```python
from build123d import *

# Parameters (mm, degrees)
SKETCH1_W           = 50
SKETCH1_H           = 60
BOSS_EXTRUDE1_DEPTH = 25
CUT_EXTRUDE1_START  = -10
SKETCH2_R           = 22.5
CUT_EXTRUDE1_DEPTH  = 30
SKETCH3_R           = 7.5
CUT_EXTRUDE2_DEPTH  = 64.442887702
SKETCH4_R           = 10
CUT_EXTRUDE3_DEPTH  = 10
SKETCH10_W          = 11
SKETCH10_H          = 10
CUT_EXTRUDE9_DEPTH  = 11
SKETCH11_R          = 2.25
CUT_EXTRUDE10_DEPTH = 50.398886748
SKETCH12_R          = 2
CUT_EXTRUDE11_DEPTH = 50.371044201
SKETCH13_R          = 3.5
CUT_EXTRUDE12_DEPTH = 50.371044201
CHAMFER1_SIZE       = 3
FILLET1_R           = 4
SKETCH14_R          = 2
CUT_EXTRUDE13_DEPTH = 10
CUT_EXTRUDE14_DEPTH = 3
BOSS_EXTRUDE2_DEPTH = 5
CHAMFER2_SIZE       = 3
FILLET2_R           = 1


with BuildPart() as part:
    # Sketch1 → Boss-Extrude1 (new body)
    with BuildSketch(Plane(origin=(0, 0, 0), x_dir=(1, 0, 0), z_dir=(0, 1, 0))):
        Rectangle(SKETCH1_W, SKETCH1_H)
    extrude(amount=BOSS_EXTRUDE1_DEPTH)

    # Sketch2 → Cut-Extrude1 (cut)
    with BuildSketch(Plane.ZY.offset(25).offset(CUT_EXTRUDE1_START)):
        with Locations((0, 25)):
            Circle(SKETCH2_R)
    extrude(amount=-CUT_EXTRUDE1_DEPTH, mode=Mode.SUBTRACT)

    # Sketch3 → Cut-Extrude2 (cut, through all)
    with BuildSketch(Plane.ZY.offset(25)):
        with Locations((0, 25)):
            Circle(SKETCH3_R)
    extrude(amount=-CUT_EXTRUDE2_DEPTH, mode=Mode.SUBTRACT)

    # Sketch4 → Cut-Extrude3 (cut)
    with BuildSketch(Plane.XY.offset(30)):
        with Locations((0, 25)):
            Circle(SKETCH4_R)
    extrude(amount=-CUT_EXTRUDE3_DEPTH, mode=Mode.SUBTRACT)

    # Sketch10 → Cut-Extrude9 (cut)
    with BuildSketch(Plane(origin=(25, 0, 0), x_dir=(0, 0, -1), z_dir=(1, 0, 0))):
        with Locations((-10, 5)):
            Rectangle(SKETCH10_W, SKETCH10_H)
        with Locations((10, 5)):
            Rectangle(SKETCH10_W, SKETCH10_H)
    cut_extrude9 = extrude(amount=-CUT_EXTRUDE9_DEPTH, mode=Mode.SUBTRACT)

    # Sketch11 → Cut-Extrude10 (cut, symmetric)
    with BuildSketch(Plane(origin=(0, 0, -4.5), x_dir=(-1, 0, 0), z_dir=(0, 0, -1))):
        with Locations(Location((-21, 5, 0), (0, 0, 90))):
            Circle(SKETCH11_R)
    cut_extrude10 = extrude(amount=CUT_EXTRUDE10_DEPTH, both=True, mode=Mode.SUBTRACT)

    # Mirror1: Cut-Extrude9, Cut-Extrude10 across plane
    add(cut_extrude9.mirror(Plane(origin=(0, 0, 0), x_dir=(0, 0, 1), z_dir=(1, 0, 0))), mode=Mode.SUBTRACT)
    add(cut_extrude10.mirror(Plane(origin=(0, 0, 0), x_dir=(0, 0, 1), z_dir=(1, 0, 0))), mode=Mode.SUBTRACT)

    # Sketch12 → Cut-Extrude11 (cut, symmetric)
    with BuildSketch(Plane(origin=(0, -2.5, 2.5), x_dir=(1, 0, 0), z_dir=(0, -0.7071067811865475, 0.7071067811865477))):
        with Locations(Location((20, 33.890872965, 0), (0, 0, 270))):
            Circle(SKETCH12_R)
        with Locations(Location((-20, 33.890872965, 0), (0, 0, 270))):
            Circle(SKETCH12_R)
    cut_extrude11 = extrude(amount=CUT_EXTRUDE11_DEPTH, both=True, mode=Mode.SUBTRACT)

    # Sketch13 → Cut-Extrude12 (cut, through all)
    with BuildSketch(Plane(origin=(0, -2.5, 2.5), x_dir=(1, 0, 0), z_dir=(0, -0.7071067811865475, 0.7071067811865477))):
        with Locations(Location((-20, 33.890872965, 0), (0, 0, 90))):
            Circle(SKETCH13_R)
        with Locations(Location((20, 33.890872965, 0), (0, 0, 90))):
            Circle(SKETCH13_R)
    cut_extrude12 = extrude(amount=CUT_EXTRUDE12_DEPTH, mode=Mode.SUBTRACT)

    # Mirror3: Cut-Extrude11, Cut-Extrude12 across plane
    add(cut_extrude11.mirror(Plane.XY), mode=Mode.SUBTRACT)
    add(cut_extrude12.mirror(Plane.XY), mode=Mode.SUBTRACT)

    # Chamfer1
    # the kernel refuses this chamfer: 3 mm, written as the material it takes off along each edge
    with BuildSketch(Plane(origin=(25, -7.715048964, -30), x_dir=(-0.9996219169112965, 0, -0.02749587661058676), z_dir=(0, 1, 0))) as chamfer1_piece_1:
        Polygon((CHAMFER1_SIZE * 0.999621916911, CHAMFER1_SIZE * 0.0274958766106), (-CHAMFER1_SIZE * 0.0274958766106, CHAMFER1_SIZE * 0.999621916911), (0, 0), align=None)
    extrude(amount=40.430097928, mode=Mode.SUBTRACT)
    with BuildSketch(Plane(origin=(-25, -7.715048964, -30), x_dir=(0.9996219169112965, 0, -0.02749587661058676), z_dir=(0, 1, 0))) as chamfer1_piece_2:
        Polygon((CHAMFER1_SIZE * 0.999621916911, -CHAMFER1_SIZE * 0.0274958766106), (-CHAMFER1_SIZE * 0.0274958766106, -CHAMFER1_SIZE * 0.999621916911), (0, 0), align=None)
    extrude(amount=40.430097928, mode=Mode.SUBTRACT)

    # Fillet1
    fillet1_edges = [part.edges().sort_by_distance(p)[0] for p in [
        (-25, 10, 10),
        (-25, 10, -10),
        (25, 10, 10),
        (25, 10, -10),
    ]]
    fillet(fillet1_edges, radius=FILLET1_R)

    # Sketch14 → Cut-Extrude13 (cut)
    with BuildSketch(Plane.XZ):
        with Locations(Location((-15, -20.205680561, 0), (0, 0, 270))):
            Circle(SKETCH14_R)
        with Locations(Location((15, -20.205680561, 0), (0, 0, 270))):
            Circle(SKETCH14_R)
    extrude(amount=-CUT_EXTRUDE13_DEPTH, mode=Mode.SUBTRACT)

    # Sketch15 → Cut-Extrude14 (cut)
    with BuildSketch(Plane.XY.offset(30)):
        Polygon((-21, 0.958548116), (-17.5, 2.979274058), (-17.5, 7.020725942), (-21, 9.041451884), (-24.5, 7.020725942), (-24.5, 2.979274058), align=None)
        Polygon((21, 0.958548116), (24.5, 2.979274058), (24.5, 7.020725942), (21, 9.041451884), (17.5, 7.020725942), (17.5, 2.979274058), align=None)
    extrude(amount=-CUT_EXTRUDE14_DEPTH, mode=Mode.SUBTRACT)

    # Sketch16 → Boss-Extrude2 (add)
    with BuildSketch(Plane.XY.offset(30)):
        with BuildLine():
            Line((-25, 9.464101615), (-27, 6))
            Line((-27, 6), (-27, 0))
            ThreePointArc((-27, 0), (-26.414213562, -1.414213562), (-25, -2))
            Line((-25, -2), (-19, -2))
            Line((-19, -2), (-15.535898385, 0))
            Line((-15.535898385, 0), (-25, 0))
            Line((-25, 0), (-25, 9.464101615))
        make_face()
    boss_extrude2 = extrude(amount=-BOSS_EXTRUDE2_DEPTH)

    # Mirror4: Boss-Extrude2 across plane
    add(boss_extrude2.mirror(Plane(origin=(0, 0, 0), x_dir=(0, 0, 1), z_dir=(1, 0, 0))))

    # Chamfer2
    # the kernel refuses this chamfer: 3 mm, written as the material it takes off along each edge
    with BuildSketch(Plane(origin=(-25, 0, 25), x_dir=(0.9996219169112968, -0.02749587661058636, 0), z_dir=(0, 0, -1))) as chamfer2_piece_1:
        Polygon((CHAMFER2_SIZE * 0.999621916911, -CHAMFER2_SIZE * 0.0274958766106), (-CHAMFER2_SIZE * 0.0274958766106, -CHAMFER2_SIZE * 0.999621916911), (0, 0), align=None)
    extrude(amount=17.215048964, mode=Mode.SUBTRACT)
    with BuildSketch(Plane(origin=(-25, 0, 12.215048964), x_dir=(0.9996219169112968, -0.02749587661058636, 0), z_dir=(0, 0, -1))) as chamfer2_piece_2:
        Polygon((CHAMFER2_SIZE * 0.999621916911, -CHAMFER2_SIZE * 0.0274958766106), (-CHAMFER2_SIZE * 0.0274958766106, -CHAMFER2_SIZE * 0.999621916911), (0, 0), align=None)
    extrude(amount=24.430097928, mode=Mode.SUBTRACT)
    with BuildSketch(Plane(origin=(-25, 0, -7.784951036), x_dir=(0.9996219169112968, -0.02749587661058636, 0), z_dir=(0, 0, -1))) as chamfer2_piece_3:
        Polygon((CHAMFER2_SIZE * 0.999621916911, -CHAMFER2_SIZE * 0.0274958766106), (-CHAMFER2_SIZE * 0.0274958766106, -CHAMFER2_SIZE * 0.999621916911), (0, 0), align=None)
    extrude(amount=26.930097928, mode=Mode.SUBTRACT)
    with BuildSketch(Plane(origin=(-16.54463656, 0, -35.45536344), x_dir=(0.7068394360709561, -0.027495876610586396, 0.7068394360703909), z_dir=(-0.7071067811862648, 0, 0.7071067811868302))) as chamfer2_piece_4:
        Polygon((CHAMFER2_SIZE * 0.999621916911, CHAMFER2_SIZE * 0.0274958766106), (-CHAMFER2_SIZE * 0.0274958766106, CHAMFER2_SIZE * 0.999621916911), (0, 0), align=None)
    extrude(amount=19.672738615, mode=Mode.SUBTRACT)
    with BuildSketch(Plane(origin=(-29.715048964, 0, -30), x_dir=(0, -0.02749587661058636, 0.9996219169112968), z_dir=(1, 0, 0))) as chamfer2_piece_5:
        Polygon((CHAMFER2_SIZE * 0.999621916911, -CHAMFER2_SIZE * 0.0274958766106), (-CHAMFER2_SIZE * 0.0274958766106, -CHAMFER2_SIZE * 0.999621916911), (0, 0), align=None)
    extrude(amount=59.430097928, mode=Mode.SUBTRACT)
    with BuildSketch(Plane(origin=(16.54463656, 0, -35.45536344), x_dir=(-0.7068394360709561, -0.027495876610586396, 0.7068394360703909), z_dir=(0.7071067811862648, 0, 0.7071067811868302))) as chamfer2_piece_6:
        Polygon((CHAMFER2_SIZE * 0.999621916911, -CHAMFER2_SIZE * 0.0274958766106), (-CHAMFER2_SIZE * 0.0274958766106, -CHAMFER2_SIZE * 0.999621916911), (0, 0), align=None)
    extrude(amount=19.672738615, mode=Mode.SUBTRACT)
    with BuildSketch(Plane(origin=(25, 0, -34.715048964), x_dir=(0.027495876610586778, 0.9996219169112968, 0), z_dir=(0, 0, 1))) as chamfer2_piece_7:
        Polygon((CHAMFER2_SIZE * 0.999621916911, CHAMFER2_SIZE * 0.0274958766106), (-CHAMFER2_SIZE * 0.0274958766106, CHAMFER2_SIZE * 0.999621916911), (0, 0), align=None)
    extrude(amount=26.930097928, mode=Mode.SUBTRACT)
    with BuildSketch(Plane(origin=(25, 0, 7.784951036), x_dir=(0.027495876610586778, 0.9996219169112968, 0), z_dir=(0, 0, 1))) as chamfer2_piece_8:
        Polygon((CHAMFER2_SIZE * 0.999621916911, CHAMFER2_SIZE * 0.0274958766106), (-CHAMFER2_SIZE * 0.0274958766106, CHAMFER2_SIZE * 0.999621916911), (0, 0), align=None)
    extrude(amount=17.215048964, mode=Mode.SUBTRACT)
    with BuildSketch(Plane(origin=(25, 0, -12.215048964), x_dir=(0.027495876610586778, 0.9996219169112968, 0), z_dir=(0, 0, 1))) as chamfer2_piece_9:
        Polygon((CHAMFER2_SIZE * 0.999621916911, CHAMFER2_SIZE * 0.0274958766106), (-CHAMFER2_SIZE * 0.0274958766106, CHAMFER2_SIZE * 0.999621916911), (0, 0), align=None)
    extrude(amount=24.430097928, mode=Mode.SUBTRACT)

    # Fillet2
    fillet2_edges = [part.edges().sort_by_distance(p)[0] for p in [
        (-18.767949192, 0, 25),
        (18.767949192, 0, 25),
        (-25, 6.232050808, 25),
        (25, 6.232050808, 25),
        (-23.5, 1.5, 25),
        (23.5, 1.5, 25),
    ]]
    fillet(fillet2_edges, radius=FILLET2_R)


solid = part.part
```
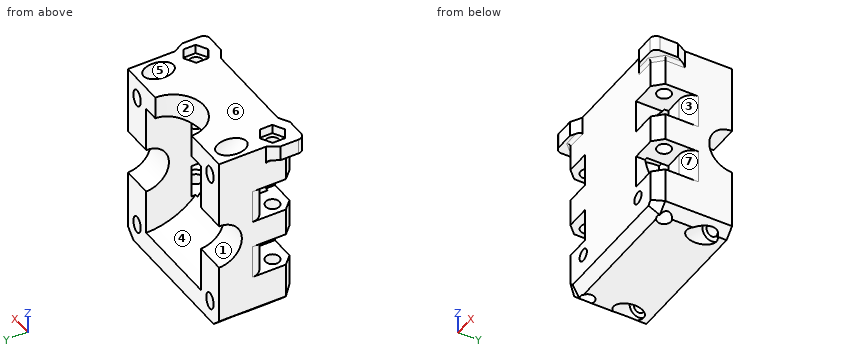
Check sheet for the modelled part. Datum: model origin and axes. Units: mm. Face numbers are marked on the shaded views. A direction names the side the tool comes from. Give positions to 0.01 mm unless a question says otherwise; leave off trailing zeros. Order: outer loops, then holes, each group sorted by start corner. A loop starts at its lowest first (then second) coordinate and runs counter-clockwise, first axis right, second up. Notation, with made-up numbers: M 20,79.5 L 76,79.5 A18 cw 76,94.5 Z; hole C 50,-33.75 d10. An arc over 180 degrees is marked long. Answer in a Markdown table with one row per item.
1) Cross-section at D-D, the plane y = 5. Count the separate pieces of the cut face and the enclosed holes in it, plus the area to 3 significant figures.
Filled sheet:
| item | result |
|---|---|
| separate pieces | 10 |
| enclosed holes | 2 |
| area | 1,550 mm2 |
2) Gauge pin test, flat ends, axial feed: P1, Ø4, axis at x = 21, y = 5, coming from the +Z side; P2, Ø8, axis at y = 9.5, z = -22, coming from the +X side; P3, Ø5, axis at x = -17, z = -8, coming from the -Y side; P4, Ø5.5, axis at x = -20.5, y = 4.5, coming from the +Z side. Record the tip position at first contact, or that the pin passes through.
Filled sheet:
| item | result |
|---|---|
| P1 | passes through |
| P2 | stops at x = 25 |
| P3 | stops at y = 10 |
| P4 | stops at z = 27 |
3) Cross-section at B-B, the plane z = -14.5. Enter the section's corners in (x, y), plus the area to 3 significant figures.
Filled sheet:
| item | result |
|---|---|
| outline | M -25,14 A4 ccw -21,10 L -15,10 L -15,25 L -25,25 Z; M -14,0 L 14,0 L 14,7.8 L -14,7.8 Z; M 15,10 L 21,10 A4 ccw 25,14 L 25,25 L 15,25 Z |
| area | 511 mm2 |
4) Cross-section at A-A, the plane x = 0. Enter the section's corners in (y, z), plus the area to 3 significant figures.
Filled sheet:
| item | result |
|---|---|
| outline | M 0,-27 L 3,-30 L 25,-30 L 25,-22.5 A22.5 cw 15,20.16 L 15,30 L 0,30 Z |
| area | 618 mm2 |
5) Cross-section at C-C, the plane z = 0. Enter the section's corners in (x, y).
Filled sheet:
| item | result |
|---|---|
| outline | M -25,3 L -22,0 L 22,0 L 25,3 L 25,17.5 L 15,17.5 L 15,2.5 L -15,2.5 L -15,17.5 L -25,17.5 Z; hole C -21,5 d4.5; hole C 21,5 d4.5 |
6) Access from +Z, -Z, +X, -X, +Y, -Y to the whole of each face (thin tool, end or side, straight path). Record for the marked faces 1, 2, 3 and 4.
Filled sheet:
| item | result |
|---|---|
| face 1 | +X, -X, +Y |
| face 2 | +Z, +Y |
| face 3 | +X, -Y |
| face 4 | +Y |
7) Thickness scan on L1, parallel to X at y = 5, z = 22.25; L2, parallel to Z at x = -18.5, y = 7.75; L3, parallel to X at y = 10.25, z = -16.5. Record the ranges inside material, lowest first. Write a range as [from, to].
Filled sheet:
| item | result |
|---|---|
| L1 | x = [-25, -23.25], [-18.75, 18.75], [23.25, 25] |
| L2 | z = [-30, -15.5], [-4.5, 4.5], [15.5, 30] |
| L3 | x = [-25, -15], [15, 25] |
8) Release check for a two-part mould opening along X. For the marked faces 5, 6 and 7 record: +X half, -X half, draft (parallel to the pull), parting line (faces both ways), or undercut.
Filled sheet:
| item | result |
|---|---|
| face 5 | undercut |
| face 6 | draft |
| face 7 | +X half |
